Read the model definition and answer for the solid it produces. Units are mm, in the model's axes. Face numbers are marked on the shaded views. Coordinates: 2 decimals unless noted, no trailing zeros. Write each loop counter-clockwise with the first axis right and the second up, starting at its lowest first coordinate (ties: lowest second). Pieces come first, ordered by that corner, then holes. Notation, with made-up numbers: (-17.5, 89.25) -> (23.5, 89.25) arc R21 ccw to (23.5, 115.25) -> close; hole circle Ø4 at (66.5, 10). An arc over 180 degrees is marked (long way). Write item = value, one per line. Start each with the question number.
1) Section C-C (x = 0) is taken. Determine the outline of the cut face in (y, z), plus the area to 3 significant figures.
2) Section B-B (y = 9) is taken. Determine the outline of the cut face in (x, z), plus the area to 3 significant figures.
3) Section D-D (z = -4) is taken. Count the separate pieces of the cut face and the enclosed holes in it, plus the area to 3 significant figures.
4) For a pull along Y with two mould halves and no side action, classify the marked faces 1, 2 and 3 as released by +Y, released by -Y, zero draft, split by the parting line, or undercut.
5) Find the intervals of material crossed by line 1 along Y through (x, z) = (-10, 5); line 2 along Y through (x, z) = (-3, -5.5); line 3 along Y through (x, z) = (1, 5.25), in increasing order. Write a range as from..to.
6) Flat-ended cylindrical pins translate along their axes: pin 1 Ø9 at (x, y) = (-10, 75) entering from -Z; pin 2 Ø10.5 at (x, y) = (0, 9) entering from +Z. Find the tip coordinate at first contact, or state that the pin passes through.
7) Section A-A (x = -10) is taken. Determine the outline of the cut face in (y, z), plus the area to 3 significant figures.
from build123d import *

# Parameters (mm, degrees)
CROQUIS1_W                     = 40
CROQUIS1_H                     = 170
SALIENTE_EXTRUIR1_DEPTH        = 6.35
TALADRO_DE_MARGEN_PARA_1_41_D  = 6.7564
TALADRO_DE_MARGEN_PARA_7_161_D = 11.90498


with BuildPart() as part:
    # Croquis1 → Saliente-Extruir1 (new, symmetric)
    with BuildSketch(Plane.XY):
        Rectangle(CROQUIS1_W, CROQUIS1_H)
    extrude(amount=SALIENTE_EXTRUIR1_DEPTH, both=True)

    # Taladro de margen para 1/41 (through all)
    with Locations(Plane.XY.offset(6.35)):
        with Locations((10, 75), (10, 35), (-10, 35), (-10, 75), (-10, -75), (-10, -35), (10, -35), (10, -75)):
            Hole(TALADRO_DE_MARGEN_PARA_1_41_D / 2)

    # Taladro de margen para 7/161 (through all)
    with Locations(Plane(origin=(0, 0, -6.35), x_dir=(-1, 0, 0), z_dir=(0, 0, -1))):
        with Locations((0, -9), (0, 9)):
            Hole(TALADRO_DE_MARGEN_PARA_7_161_D / 2)


solid = part.part
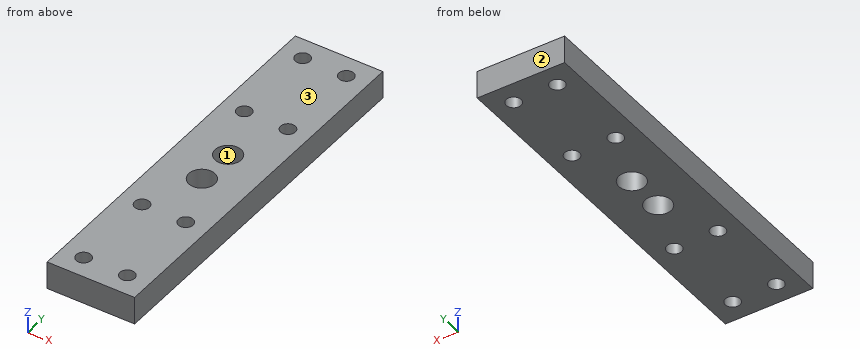
Answer key:
q1.outline = (-85, -6.35) -> (-14.95, -6.35) -> (-14.95, 6.35) -> (-85, 6.35) -> close; (-3.05, -6.35) -> (3.05, -6.35) -> (3.05, 6.35) -> (-3.05, 6.35) -> close; (14.95, -6.35) -> (85, -6.35) -> (85, 6.35) -> (14.95, 6.35) -> close
q1.area = 1,860 mm^2
q2.outline = (-20, -6.35) -> (-5.95, -6.35) -> (-5.95, 6.35) -> (-20, 6.35) -> close; (5.95, -6.35) -> (20, -6.35) -> (20, 6.35) -> (5.95, 6.35) -> close
q2.area = 357 mm^2
q3.separate_pieces = 1
q3.enclosed_holes = 10
q3.area = 6,290 mm^2
q4.face_1 = undercut
q4.face_2 = released by +Y
q4.face_3 = zero draft
q5.line_1 = -85..-78.38, -71.62..-38.38, -31.62..31.62, 38.38..71.62, 78.38..85
q5.line_2 = -85..-14.14, -3.86..3.86, 14.14..85
q5.line_3 = -85..-14.87, -3.13..3.13, 14.87..85
q6.pin_1 = -6.35
q6.pin_2 = through
q7.outline = (-85, -6.35) -> (-78.38, -6.35) -> (-78.38, 6.35) -> (-85, 6.35) -> close; (-71.62, -6.35) -> (-38.38, -6.35) -> (-38.38, 6.35) -> (-71.62, 6.35) -> close; (-31.62, -6.35) -> (31.62, -6.35) -> (31.62, 6.35) -> (-31.62, 6.35) -> close; (38.38, -6.35) -> (71.62, -6.35) -> (71.62, 6.35) -> (38.38, 6.35) -> close; (78.38, -6.35) -> (85, -6.35) -> (85, 6.35) -> (78.38, 6.35) -> close
q7.area = 1,820 mm^2
